Autodesk Inventor part; units mm, degrees
ref_plane "YZ Plane" through (0, 0, 0) normal (1, 0, 0) x (0, 1, 0)
ref_plane "XZ Plane" through (0, 0, 0) normal (0, 1, 0) x (-1, 0, 0)
ref_plane "XY Plane" through (0, 0, 0) normal (0, 0, 1) x (1, 0, 0)
sketch "Sketch1" plane through (0, 0, 0) normal (0, 1, 0) x (-1, 0, 0)
  line L0 (-110.556, -67.8158) -> (-459.806, -67.8158)
  line L1 (-459.806, -67.8158) -> (-459.806, -296.4158)
  line L2 (-459.806, -296.4158) -> (-110.556, -296.4158)
  line L3 (-110.556, -296.4158) -> (-110.556, -67.8158)
  point P0 (0, 0)
  dimension "d0" = 349.25
  dimension "d1" = 228.6
extrude "Extrusion2" add sketch "Sketch1" along normal blind 177.8
sketch "Sketch2" plane through (0, 177.8, 0) normal (0, 1, 0) x (1, 0, 0)
  arc A0 (459.806, 271.0158) -> (459.806, 93.2158) centre (470.8722, 182.1158) ccw
  line L0 (459.806, 271.0158) -> (459.806, 93.2158)
  line L1 (459.806, 67.8158) -> (459.806, 296.4158)
  point P0 (0, 0)
extrude "Extrusion3" cut sketch "Sketch2" against normal through all
sketch "Sketch3" plane through (0, 177.8, 0) normal (0, 1, 0) x (1, 0, 0)
  line L0 (110.556, 296.4158) -> (110.556, 67.8158)
  line L1 (459.806, 296.4158) -> (110.556, 296.4158)
  point P0 (0, 0)
  point P1 (199.456, 182.1158)
hole "Hole3" at (199.456, 177.8, -182.1158) direction (0, -1, 0) diameter 146.05 depth 50.8
sketch "Sketch4" plane through (199.456, 127, -182.1158) normal (0, 1, 0) x (1, 0, 0)
  point P0 (-199.456, -182.1158)
  point P1 (0, 0)
hole "Hole5" at (199.456, 127, -182.1158) direction (0, -1, 0) diameter 73.025 end through all
sketch "Sketch5" plane through (0, 177.8, 0) normal (0, 1, 0) x (1, 0, 0)
  circle A0 centre (199.456, 182.1158) radius 36.5125
  line L0 (199.456, 218.6283) -> (389.0644, 218.6283)
  arc A1 (459.806, 271.0158) -> (459.806, 93.2158) centre (470.8722, 182.1158) ccw
  line L1 (199.456, 145.6033) -> (389.0644, 145.6033)
  arc A2 (199.456, 145.6033) -> (199.456, 218.6283) centre (199.456, 182.1158) ccw
  arc A3 (389.0644, 218.6283) -> (389.0644, 145.6033) centre (470.8722, 182.1158) ccw
  point P0 (0, 0)
extrude "Extrusion5" cut sketch "Sketch5" against normal blind 101.6 contours A0 L0 A1 L1
properties part number "7.2 Part 2"
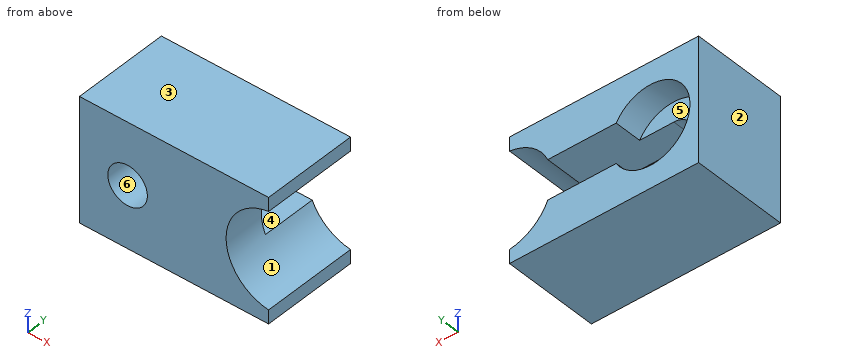
Can you work these out from the model? Positions are in its coordinate system, mm. Face numbers are marked on the shaded views. A direction names the side the tool comes from. Round coordinates to 2 decimals unless told otherwise and drop trailing zeros. Loops run counter-clockwise (first coordinate to the right, second up) from the corner with the lowest first, then second, coordinate; pieces in that order, holes last.
Item 1: Suppose I cut it at C-C, the plane y = 29.5. Write out the boundary of the cut face in (x, z) (1 decimal).
Item 2: Suppose I cut it at D-D, the plane x = 416.5. Write out the boundary of the cut face in (y, z), then the cut area to 3 significant figures.
Item 3: Suppose I cut it at B-B, the plane z = -189.5. Write out the boundary of the cut face in (x, y), then the cut area to 3 significant figures.
Item 4: Which directions (+Z, -Z, +X, -X, +Y, -Y) give clear straight access to the entire face, cutting with the end or side of a thin tool? Please do the marked faces 4, 5 and 6.
Item 5: Will these pins go through, and if not, where does the flat tip stop? pin 1 Ø10 at (y, z) = (20.5, -219) entering from +X; pin 2 Ø1.5 at (x, z) = (232.5, -240.5) entering from -Y.
Item 6: If we mould it in two halves opening along Z, with no side actions, what happens to the marked faces 1, 2 and 3? For each: +Z half, -Z half, draft (parallel to the pull), parting line (faces both ways), or undercut.
Item 7: Please list where these lines run through material, in increasing order: L1, parallel to Z at x = 304, y = 110.5; L2, parallel to X at y = 71, z = -180.5; L3, parallel to Z at x = 201.5, y = 47.
Item 8: Suppose I cut it at A-A, the plane x = 353. Write out the boundary of the cut face in (y, z).
Reported:
1. outline: (110.6, -296.4) - (459.8, -296.4) - (459.8, -271) arc R89.6 cw to (459.8, -93.2) - (459.8, -67.8) - (110.6, -67.8) - close; hole circle Ø73 at (199.5, -182.1)
2. outline: (0, -296.42) - (177.8, -296.42) - (177.8, -253.32) - (0, -253.32) - close; (0, -110.92) - (177.8, -110.92) - (177.8, -67.82) - (0, -67.82) - close
2. area: 15,300 mm2
3. outline: (110.56, 0) - (163.7, 0) - (163.7, 127) - (126.81, 127) - (126.81, 177.8) - (110.56, 177.8) - close; (235.21, 0) - (381.59, 0) - (381.59, 76.2) - (235.21, 76.2) - close
3. area: 18,700 mm2
4. face 4: +X, +Y
4. face 5: +Y
4. face 6: +Y, -Y
5. pin 1: stops at x = 391.68
5. pin 2: stops at y = 0
6. face 1: undercut
6. face 2: draft
6. face 3: +Z half
7. L1: z = -296.42 to -218.63, -145.6 to -67.82
7. L2: x = 110.56 to 162.98, 235.93 to 381.3
7. L3: z = -296.42 to -218.57, -145.66 to -67.82
8. outline: (0, -296.42) - (177.8, -296.42) - (177.8, -218.63) - (76.2, -218.63) - (76.2, -145.6) - (177.8, -145.6) - (177.8, -67.82) - (0, -67.82) - close
